from build123d import *

# Parameters (mm, degrees)
SKETCH2_R           = 14.2875
SKETCH2_R_2         = 3.175
SKETCH2_R_3         = 11.000000098
SKETCH2_R_4         = 11.1125
BOSS_EXTRUDE1_DEPTH = 6.35
CUT_EXTRUDE1_DEPTH  = 432.327965994
SKETCH4_R           = 2.4892
CUT_EXTRUDE2_DEPTH  = 432.327965994


with BuildPart() as part:
    # Sketch2 → Boss-Extrude1 (new body)
    with BuildSketch(Plane(origin=(0, 0, 0), x_dir=(1, 0, 0), z_dir=(0, 1, 0))):
        with BuildLine():
            Line((239.638116078, 289.551831635), (252.063037476, 130.700241744))
            ThreePointArc((252.063037476, 130.700241744), (255.941769276, 120.588679828), (264.705030265, 114.225229381))
            ThreePointArc((264.705030265, 114.225229381), (295.185030265, 71.12), (264.705030265, 28.014770619))
            ThreePointArc((264.705030265, 28.014770619), (249.169215503, 17.673987821), (240.408185929, 1.19558711))
            Line((240.408185929, 1.19558711), (214.878590493, -102.576218058))
            ThreePointArc((214.878590493, -102.576218058), (197.553145093, -114.543453333), (183.588238686, -98.783784318))
            Line((183.588238686, -98.783784318), (183.588238686, 55.786275092))
            ThreePointArc((183.588238686, 55.786275092), (180.651328593, 67.642479874), (172.519766888, 76.756904539))
            ThreePointArc((172.519766888, 76.756904539), (162.968469926, 90.879304348), (165.661306265, 107.714329816))
            ThreePointArc((165.661306265, 107.714329816), (170.989832116, 127.147303909), (165.661306265, 146.580278002))
            ThreePointArc((165.661306265, 146.580278002), (162.419786372, 158.402003909), (165.661306265, 170.223729816))
            ThreePointArc((165.661306265, 170.223729816), (170.989832116, 189.656703909), (165.661306265, 209.089678002))
            ThreePointArc((165.661306265, 209.089678002), (162.771672921, 224.934819973), (170.904796514, 238.837007052))
            ThreePointArc((170.904796514, 238.837007052), (184.60593815, 258.315476471), (186.286318241, 282.07065224))
            ThreePointArc((186.286318241, 282.07065224), (208.98517415, 314.173400291), (239.638116078, 289.551831635))
        make_face()
        with Locations(Location((185.597286372, 95.892603909, 0), (0, 0, 270))):
            Circle(SKETCH2_R, mode=Mode.SUBTRACT)
        with Locations(Location((185.597286372, 158.402003909, 0), (0, 0, 270))):
            Circle(SKETCH2_R, mode=Mode.SUBTRACT)
        with Locations(Location((185.597286372, 220.911403909, 0), (0, 0, 270))):
            Circle(SKETCH2_R, mode=Mode.SUBTRACT)
        with Locations(Location((212.73279296, 287.447373473, 0), (0, 0, 270))):
            Circle(SKETCH2_R, mode=Mode.SUBTRACT)
        with Locations(Location((199.463238686, -98.783784318, 0), (0, 0, 270))):
            Circle(SKETCH2_R_2, mode=Mode.SUBTRACT)
        with Locations(Location((249.465030265, 71.12, 0), (0, 0, 270))):
            Circle(SKETCH2_R_3, mode=Mode.SUBTRACT)
        with Locations(Location((226.06, 25.4, 0), (0, 0, 270))):
            Circle(SKETCH2_R_4, mode=Mode.SUBTRACT)
    extrude(amount=BOSS_EXTRUDE1_DEPTH)

    # Sketch3 → Cut-Extrude1 (cut, through all)
    with BuildSketch(Plane(origin=(0, 6.35, 0), x_dir=(1, 0, 0), z_dir=(0, 1, 0))):
        with BuildLine():
            ThreePointArc((233.536357361, 73.079561051), (235.010141069, 74.055758562), (234.033943558, 75.529542271))
            ThreePointArc((234.033943558, 75.529542271), (232.56015985, 74.553344759), (233.536357361, 73.079561051))
        make_face()
        with BuildLine():
            ThreePointArc((254.795860629, 57.173540539), (253.32207692, 56.197343028), (254.298274432, 54.72355932))
            ThreePointArc((254.298274432, 54.72355932), (255.77205814, 55.699756831), (254.795860629, 57.173540539))
        make_face()
        with BuildLine():
            ThreePointArc((264.896116972, 66.710457729), (266.369900681, 67.686655241), (265.393703169, 69.160438949))
            ThreePointArc((265.393703169, 69.160438949), (263.919919461, 68.184241438), (264.896116972, 66.710457729))
        make_face()
        with BuildLine():
            ThreePointArc((259.814079708, 81.8819078), (261.287863416, 82.858105311), (260.311665905, 84.331889019))
            ThreePointArc((260.311665905, 84.331889019), (258.837882196, 83.355691508), (259.814079708, 81.8819078))
        make_face()
        with BuildLine():
            ThreePointArc((244.134199902, 85.066459461), (245.60798361, 86.042656972), (244.631786099, 87.51644068))
            ThreePointArc((244.631786099, 87.51644068), (243.158002391, 86.540243169), (244.134199902, 85.066459461))
        make_face()
        with BuildLine():
            ThreePointArc((239.115980823, 60.3580922), (237.642197115, 59.381894689), (238.618394626, 57.908110981))
            ThreePointArc((238.618394626, 57.908110981), (240.092178334, 58.884308492), (239.115980823, 60.3580922))
        make_face()
    extrude(amount=-CUT_EXTRUDE1_DEPTH, mode=Mode.SUBTRACT)

    # Sketch4 → Cut-Extrude2 (cut, through all)
    with BuildSketch(Plane(origin=(0, 6.35, 0), x_dir=(1, 0, 0), z_dir=(0, 1, 0))):
        with Locations(Location((231.78279296, 242.997373473, 0), (0, 0, 270))):
            Circle(SKETCH4_R)
        with Locations(Location((211.334459224, 192.197373473, 0), (0, 0, 270))):
            Circle(SKETCH4_R)
        with Locations(Location((236.734459224, 179.690730842, 0), (0, 0, 270))):
            Circle(SKETCH4_R)
        with Locations(Location((211.334459224, 128.697373473, 0), (0, 0, 270))):
            Circle(SKETCH4_R)
        with Locations(Location((211.334459224, 71.547373473, 0), (0, 0, 270))):
            Circle(SKETCH4_R)
        with Locations(Location((221.688238686, -27.663784318, 0), (0, 0, 270))):
            Circle(SKETCH4_R)
        with Locations(Location((189.938238686, -60.683784318, 0), (0, 0, 270))):
            Circle(SKETCH4_R)
        with Locations(Location((277.224046368, 93.345, 0), (0, 0, 270))):
            Circle(SKETCH4_R)
        with Locations(Location((277.224046368, 48.895, 0), (0, 0, 270))):
            Circle(SKETCH4_R)
        with Locations(Location((240.695792235, 129.045416737, 0), (0, 0, 270))):
            Circle(SKETCH4_R)
    extrude(amount=-CUT_EXTRUDE2_DEPTH, mode=Mode.SUBTRACT)


solid = part.part
Can you work these out from the model? Positions are in its coordinate system, mm. Round coordinates to 2 decimals unless told otherwise and drop trailing zeros. Write item = value, one per line. Start each with the question number.
(1) If we mould it in two halves opening along X, with no side actions, what happens to faces 1 (the face through (260.37, 3.13, -72.55)), 2 (the face through (215, 6.35, -103)), 3 (the face through (163.023, 3.131, -90.641))? For each: released by +X, released by -X, zero draft, split by the parting line, or undercut.
(2) If we section it at A-A (y = 2): Give the number of separate pieces and of enclosed holes in the cut face, and give its area (3 significant figures).
(3) If I drill on probe 1 along X at (y, z) = (2.5, -71.12); probe 2 along Z at (x, y) = (196, 1.25); probe 3 along Z at (x, y) = (180.5, 3.75), over which ranges is the centre line in solid material (lowest first)? Write a range as [from, to].
(4) For P1, Ø1, axis at y = 1.5, z = -144.5, coming from the -X side; P2, Ø1.5, axis at x = 231.5, y = 3.5, coming from the -Z side; P3, Ø1, axis at y = 1.5, z = -85.5, coming from the +X side; P4, Ø13.5, axis at x = 226.06, z = -25.4, coming from the -Y side, each with a flat end and sliding along its axis, tell me the tip position at first contact or that it passes through.
Ans:
q1.face_1 = undercut
q1.face_2 = zero draft
q1.face_3 = released by -X
q2.separate_pieces = 1
q2.enclosed_holes = 23
q2.area = 26,800 mm²
q3.probe_1 = [178.44, 208.88], [213.79, 238.47], [260.47, 295.19]
q3.probe_2 = [-308.62, -230.71], [-211.12, -168.2], [-148.61, -105.69], [-86.1, 114.28]
q3.probe_3 = [-249.78, -234.26], [-207.56, -171.75], [-145.05, -109.24], [-82.55, -67.92]
q4.P1 = 166.55
q4.P2 = -307.54
q4.P3 = 293.03
q4.P4 = through
